```python
from build123d import *

# Parameters (mm, degrees)
F0_W     = 550
F0_H     = 550
F1_DEPTH = 35
F2_W     = 50
F2_H     = 50
F3_DEPTH = 450


with BuildPart() as f1:
    # F0 (on Top) → F1 (new body)
    with BuildSketch(Plane.XY):
        Rectangle(F0_W, F0_H)
    extrude(amount=-F1_DEPTH)

    # F2 (on Top) → F3 (join)
    with BuildSketch(Plane.XY):
        with Locations((250, 250)):
            Rectangle(F2_W, F2_H)
        with Locations((250, -250)):
            Rectangle(F2_W, F2_H)
        with Locations((-250, 250)):
            Rectangle(F2_W, F2_H)
        with Locations((-250, -250)):
            Rectangle(F2_W, F2_H)
    extrude(amount=-F3_DEPTH)


solid = f1.part
```
Build history of the part. All positions in model axes, mm. A direction names the side the tool comes from. Round coordinates to 2 decimals unless told otherwise and drop trailing zeros. Order: outer loops, then holes, each group sorted by start corner. A loop starts at its lowest first (then second) coordinate and runs counter-clockwise, first axis right, second up. Notation, with made-up numbers: (17, 3) -> (26, 3) arc R24 ccw to (26, 18) -> close; hole circle Ø9 at (59, 17.25). An arc over 180 degrees is marked (long way). Answer in a Markdown table with one row per item.
1) Wall check: L1, parallel to Z at x = 216, y = -162; L2, parallel to Y at x = 239, z = -108. Give the ranges that are in metal, low to high.
Values:
| item | result |
|---|---|
| L1 | -35 to 0 |
| L2 | -275 to -225, 225 to 275 |
2) Band-saw the part on A-A on z = -107. Give the cut face in (x, y), and give its area (3 significant figures).
Values:
| item | result |
|---|---|
| outline | (-275, -275) -> (-225, -275) -> (-225, -225) -> (-275, -225) -> close; (-275, 225) -> (-225, 225) -> (-225, 275) -> (-275, 275) -> close; (225, -275) -> (275, -275) -> (275, -225) -> (225, -225) -> close; (225, 225) -> (275, 225) -> (275, 275) -> (225, 275) -> close |
| area | 10,000 mm2 |
3) Pin check, flat tip, straight feed: P1, Ø2, axis at x = 72.5, y = -113, coming from the -Z side. Stop position of the tip, or through.
Values:
| item | result |
|---|---|
| P1 | z = -35 |
4) Mould opens along X. For faces 4 (the flat face through (-275, -42, -7)), 5 (the flat face through (-42, 275, -7)), 6 (the flat face through (275, -42, -7)), 7 (the flat face through (225, -250, -240)) say: released by +X, released by -X, zero draft, split by the parting line, or undercut.
Values:
| item | result |
|---|---|
| face 4 | released by -X |
| face 5 | zero draft |
| face 6 | released by +X |
| face 7 | undercut |
5) Band-saw the part on B-B on x = -22. Give the cut face in (y, z), and give its area (4 significant figures).
Values:
| item | result |
|---|---|
| outline | (-275, -35) -> (275, -35) -> (275, 0) -> (-275, 0) -> close |
| area | 19,250 mm2 |
6) Which spindle directions (+Z, -Z, +X, -X, +Y, -Y) get a long thin tool onto all of the face, cutting with end or side? Do faces 1 (the flat face through (250, -225, -240)), 2 (the flat face through (-225, -250, -240)), 3 (the flat face through (250, -250, -450)). Say none if no direction does.
Values:
| item | result |
|---|---|
| face 1 | -Z, +X, -X |
| face 2 | -Z, +Y, -Y |
| face 3 | -Z, +X, -X, +Y, -Y |
